The listing builds one solid part. Answer for the finished solid, in the listing's coordinates (mm). Coordinates: 2 decimals unless noted, no trailing zeros. Write each loop counter-clockwise with the first axis right and the second up, starting at its lowest first coordinate (ties: lowest second). Pieces come first, ordered by that corner, then holes. Notation, with made-up numbers: M 12,4 L 30,4 A24 cw 30,22 Z; hole C 11,18 d6. An arc over 180 degrees is marked long. Answer as a JSON object with one key per item and string values. Group by question number.
from build123d import *

# Parameters (mm, degrees)
SKETCH1_W           = 623.55984
SKETCH1_H           = 78.16342
BASE_FLANGE1_DEPTH  = 1.5875
SKETCH3_R           = 2.75
SKETCH3_R_2         = 2.921
SKETCH3_W           = 32.08
SKETCH3_H           = 32.08
CUT_EXTRUDE3_DEPTH  = 389.990867909
SKETCH6_W           = 623.55984
SKETCH6_H           = 13.4112
BOSS_EXTRUDE1_DEPTH = 1.5875


# Sheet-metal steps are written as plain solids
with BuildPart() as part:
    # Sketch1 → Base-Flange1 (new body)
    with BuildSketch(Plane.XY):
        with Locations((-38.857061865, -129.337653818)):
            Rectangle(SKETCH1_W, SKETCH1_H)
    extrude(amount=-BASE_FLANGE1_DEPTH)

    # Sketch3 → Cut-Extrude3 (cut, through all)
    with BuildSketch(Plane.XY):
        with Locations((92.914515529, -110.369060902)):
            Circle(SKETCH3_R)
        with Locations((35.391947046, -147.147547142)):
            Circle(SKETCH3_R_2)
        with Locations((-169.771284735, -114.165270711)):
            Circle(SKETCH3_R_2)
        with Locations((-223.149152531, -156.736460083)):
            Circle(SKETCH3_R_2)
        with Locations((-304.149901865, -121.952427932)):
            Rectangle(SKETCH3_W, SKETCH3_H)
        with Locations((-86.931641865, -121.952427932)):
            Rectangle(SKETCH3_W, SKETCH3_H)
        with Locations((12.392518135, -121.952427932)):
            Rectangle(SKETCH3_W, SKETCH3_H)
        with Locations((229.610778135, -121.952427932)):
            Rectangle(SKETCH3_W, SKETCH3_H)
    extrude(amount=-CUT_EXTRUDE3_DEPTH, mode=Mode.SUBTRACT)

    # Sketch6 → Boss-Extrude1 (add, through all)
    with BuildSketch(Plane.XY):
        with Locations((-38.857061865, -83.550343818)):
            Rectangle(SKETCH6_W, SKETCH6_H)
    extrude(amount=-BOSS_EXTRUDE1_DEPTH)


solid = part.part
Item 1: Flat-ended cylindrical pins translate along their axes: pin 1 Ø3.5 at (x, y) = (92.91, -110.37) entering from -Z; pin 2 Ø6 at (x, y) = (-16, -119) entering from +Z. Find the tip coordinate at first contact, or state that the pin passes through.
Item 2: A cutting plane is placed at C-C, the plane z = -0.35. State how many separate pieces and enclosed holes the cut face has, and give its area (3 significant figures).
Item 3: Consider L1, parallel to X at y = -128, z = -0.25; L2, parallel to X at y = -108, z = -1.2; L3, parallel to X at y = -109, z = -1.3. Determine where each line is inside the solid, lowest interval first. Write a range as from..to.
Item 4: A cutting plane is placed at A-A, the plane y = -130. Write down the section's boundary in (x, z), and give its area (3 significant figures).
Item 5: A cutting plane is placed at B-B, the plane x = 8. Write down the section's boundary in (y, z).
Answer:
{
 "1": {"pin 1": "through", "pin 2": "z = 0"},
 "2": {"separate pieces": "1", "enclosed holes": "8", "area": "52,900 mm2"},
 "3": {"L1": "-350.64..-320.19, -288.11..-102.97, -70.89..-3.65, 28.43..213.57, 245.65..272.92", "L2": "-350.64..-320.19, -288.11..-102.97, -70.89..-3.65, 28.43..91.52, 94.31..213.57, 245.65..272.92", "L3": "-350.64..-320.19, -288.11..-102.97, -70.89..-3.65, 28.43..90.53, 95.3..213.57, 245.65..272.92"},
 "4": {"outline": "M -350.64,-1.59 L -320.19,-1.59 L -320.19,0 L -350.64,0 Z; M -288.11,-1.59 L -102.97,-1.59 L -102.97,0 L -288.11,0 Z; M -70.89,-1.59 L -3.65,-1.59 L -3.65,0 L -70.89,0 Z; M 28.43,-1.59 L 213.57,-1.59 L 213.57,0 L 28.43,0 Z; M 245.65,-1.59 L 272.92,-1.59 L 272.92,0 L 245.65,0 Z", "area": "786 mm2"},
 "5": {"outline": "M -168.42,-1.59 L -137.99,-1.59 L -137.99,0 L -168.42,0 Z; M -105.91,-1.59 L -76.84,-1.59 L -76.84,0 L -105.91,0 Z"}
}
